Can you work these out from the model? Positions are in its coordinate system, mm. Face numbers are marked on the shaded views. A direction names the side the tool comes from. Coordinates: 2 decimals unless noted, no trailing zeros. Write each loop counter-clockwise with the first axis right and the second up, starting at its lowest first coordinate (ties: lowest second). Pieces come first, ordered by that corner, then holes. Notation, with made-up numbers: (8.25, -25) -> (58.25, -25) arc R9 ccw to (58.25, -14) -> close; hole circle Ø9 at (1, -10.75). An arc over 180 degrees is marked (long way). Use one line per item in the form item = value.
```python
from build123d import *

# Parameters (mm, degrees)
SKETCH1_R           = 1.3
BOSS_EXTRUDE1_DEPTH = 3
SKETCH2_W           = 3
SKETCH2_H           = 32
BOSS_EXTRUDE2_DEPTH = 22
BOSS_EXTRUDE3_START = 3
BOSS_EXTRUDE3_DEPTH = 3
SKETCH7_R           = 2.5
SKETCH7_R_2         = 1.3
CUT_EXTRUDE1_DEPTH  = 3


with BuildPart() as part:
    # Sketch1 → Boss-Extrude1 (new body)
    # profile 1 of 3: a face of its own
    with BuildSketch(Plane(origin=(0, 0, 0), x_dir=(1, 0, 0), z_dir=(0, 1, 0))):
        with BuildLine():
            Line((11, -60), (11, 0))
            ThreePointArc((11, 0), (0, -11), (-11, 0))
            Line((-11, 0), (-11, -60))
            Line((-11, -60), (11, -60))
        make_face()
    # profile 2 of 3: a face of its own
    with BuildSketch(Plane(origin=(0, 0, 0), x_dir=(1, 0, 0), z_dir=(0, 1, 0))):
        with BuildLine():
            Line((11, 0), (9.3, 0))
            ThreePointArc((9.3, 0), (8, -1.3), (6.7, 0))
            Line((6.7, 0), (5, 0))
            ThreePointArc((5, 0), (0, -5), (-5, 0))
            Line((-5, 0), (-6.7, 0))
            ThreePointArc((-6.7, 0), (-8, -1.3), (-9.3, 0))
            Line((-9.3, 0), (-11, 0))
            ThreePointArc((-11, 0), (0, -11), (11, 0))
        make_face()
        with Locations(Location((0, -8, 0), (0, 0, 270))):
            Circle(SKETCH1_R, mode=Mode.SUBTRACT)
    # profile 3 of 3: a face of its own
    with BuildSketch(Plane(origin=(0, 0, 0), x_dir=(1, 0, 0), z_dir=(0, 1, 0))):
        with BuildLine():
            ThreePointArc((6.7, 0), (8, 1.3), (9.3, 0))
            Line((9.3, 0), (11, 0))
            ThreePointArc((11, 0), (0, 11), (-11, 0))
            Line((-11, 0), (-9.3, 0))
            ThreePointArc((-9.3, 0), (-8, 1.3), (-6.7, 0))
            Line((-6.7, 0), (-5, 0))
            ThreePointArc((-5, 0), (0, 5), (5, 0))
            Line((5, 0), (6.7, 0))
        make_face()
        with Locations(Location((0, 8, 0), (0, 0, 270))):
            Circle(SKETCH1_R, mode=Mode.SUBTRACT)
    extrude(amount=BOSS_EXTRUDE1_DEPTH)

    # Sketch2 → Boss-Extrude2 (add)
    with BuildSketch(Plane(origin=(11, 0, 0), x_dir=(0, 0, -1), z_dir=(1, 0, 0))):
        with Locations((-65.5, -20)):
            Rectangle(SKETCH2_W, SKETCH2_H)
        with BuildLine():
            ThreePointArc((-60, 3), (-64.949747468, 0.949747468), (-67, -4))
            Line((-67, -4), (-64, -4))
            ThreePointArc((-64, -4), (-62.828427125, -1.171572875), (-60, 0))
            Line((-60, 0), (-60, 3))
        make_face()
        with BuildLine():
            ThreePointArc((-64, -36), (-62.828427125, -38.828427125), (-60, -40))
            Line((-60, -40), (-60, -43))
            ThreePointArc((-60, -43), (-64.949747468, -40.949747468), (-67, -36))
            Line((-67, -36), (-64, -36))
        make_face()
    extrude(amount=-BOSS_EXTRUDE2_DEPTH)

    # Sketch6 → Boss-Extrude3 (add)
    with BuildSketch(Plane(origin=(0, -40, 0), x_dir=(-1, 0, 0), z_dir=(0, -1, 0)).offset(BOSS_EXTRUDE3_START)):
        with BuildLine():
            Line((11, -60), (11, 0))
            ThreePointArc((11, 0), (0, -11), (-11, 0))
            Line((-11, 0), (-11, -60))
            Line((-11, -60), (11, -60))
        make_face()
        with BuildLine():
            ThreePointArc((-5, 0), (0, 5), (5, 0))
            Line((5, 0), (11, 0))
            ThreePointArc((11, 0), (0, 11), (-11, 0))
            Line((-11, 0), (-5, 0))
        make_face()
        with BuildLine():
            Line((11, 0), (5, 0))
            ThreePointArc((5, 0), (0, -5), (-5, 0))
            Line((-5, 0), (-11, 0))
            ThreePointArc((-11, 0), (0, -11), (11, 0))
        make_face()
    extrude(amount=-BOSS_EXTRUDE3_DEPTH)

    # Sketch7 → Cut-Extrude1 (cut)
    with BuildSketch(Plane.XY.offset(67)):
        with Locations((0, -20)):
            Circle(SKETCH7_R)
        with Locations((5, -20)):
            Circle(SKETCH7_R_2)
        with Locations((-5, -20)):
            Circle(SKETCH7_R_2)
        with Locations((0, -25)):
            Circle(SKETCH7_R_2)
        with Locations((0, -15)):
            Circle(SKETCH7_R_2)
    extrude(amount=-CUT_EXTRUDE1_DEPTH, mode=Mode.SUBTRACT)


solid = part.part
```
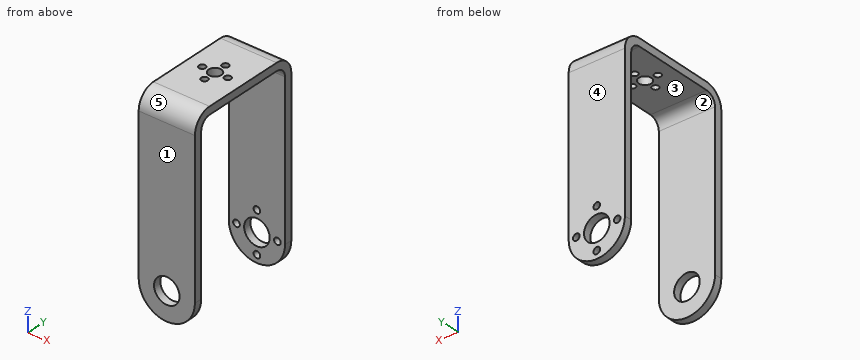
Q1. Suppose I cut it at C-C (x = 7.5). Write out the boundary of the cut face in (y, z), then the cut area to 3 significant figures.
Return value:
outline = (-43, -8.05) -> (-40, -8.05) -> (-40, 60) arc R4 cw to (-36, 64) -> (-4, 64) arc R4 cw to (0, 60) -> (0, 1.2) -> (3, 1.2) -> (3, 60) arc R7 ccw to (-4, 67) -> (-36, 67) arc R7 ccw to (-43, 60) -> close; (0, -8.05) -> (3, -8.05) -> (3, -1.2) -> (0, -1.2) -> close
area = 549 mm2
Q2. Suppose I cut it at B-B (y = -15). Write out the boundary of the cut face in (x, z).
Return value:
outline = (-11, 64) -> (-1.3, 64) -> (-1.3, 67) -> (-11, 67) -> close; (1.3, 64) -> (11, 64) -> (11, 67) -> (1.3, 67) -> close
Q3. Thinking about a two-plate mould opening in Z: for the marked faces 3, 4 and 5, which applies, released by +Z, released by -Z, zero draft, split by the parting line, or undercut?
Return value:
face_3 = released by -Z
face_4 = zero draft
face_5 = released by +Z
Q4. Suppose I cut it at D-D (z = -8). Write out the boundary of the cut face in (x, y), then the cut area to 3 significant figures.
Return value:
outline = (-7.55, -43) -> (7.55, -43) -> (7.55, -40) -> (-7.55, -40) -> close; (-7.55, 0) -> (-1.3, 0) -> (-1.3, 3) -> (-7.55, 3) -> close; (1.3, 0) -> (7.55, 0) -> (7.55, 3) -> (1.3, 3) -> close
area = 82.8 mm2
Q5. Suppose I cut it at A-A (z = 46). Write out the boundary of the cut face in (x, y).
Return value:
outline = (-11, -43) -> (11, -43) -> (11, -40) -> (-11, -40) -> close; (-11, 0) -> (11, 0) -> (11, 3) -> (-11, 3) -> close
Q6. If I drill on line 1 (Y direction, x = 6.75, z = 6); line 2 (Y direction, x = 5, z = 65.75); line 3 (Y direction, x = 0, z = 65.4), over which ranges is the centre line in solid material (lowest first)? Write a range as from..to.
Return value:
line_1 = -43..-40, 0..3
line_2 = -39.99..-21.3, -18.7..-0.01
line_3 = -40.45..-26.3, -23.7..-22.5, -17.5..-16.3, -13.7..0.45
Q7. Will these pins go through, and if not, where does the flat tip stop? pin 1 (2.5 mm diameter, centred on x = -8, z = 0, fed in from +Y); pin 2 (6.5 mm diameter, centred on x = 3, y = -20, fed in from -Z).
Return value:
pin_1 = -40
pin_2 = 64
Q8. For the marked faces 1 and 2, which set-ups out of +Z, -Z, +X, -X, +Y, -Y let a thin tool reach every point of the face, with its end or its side?
Return value:
face_1 = +Z, -Z, +X, -X, -Y
face_2 = -Z, +X, -X
